Input: part model. Units: mm. Frame: model coordinates. Face numbers are marked on the shaded views. Round coordinates to 2 decimals unless told otherwise and drop trailing zeros. Loops run counter-clockwise (first coordinate to the right, second up) from the corner with the lowest first, then second, coordinate; pieces in that order, holes last. Notation, with made-up numbers: (34.25, -35) -> (63.25, -35) arc R11 cw to (63.25, -30) -> close; hole circle Ø7 at (37.25, 25.5). An arc over 180 degrees is marked (long way). Answer as a JSON object with one key per item and string values. Group by question number.
Item 1: Material intervals for line 1 (X direction, y = 34.5, z = 0); line 2 (X direction, y = 37.5, z = -2); line 3 (Z direction, x = -2.5, y = 18.5), sorted ascending. Write a range as [from, to].
Item 2: Draft query along Z for the marked faces 1, 2, 3 and 4. Return one class per face: released by +Z, released by -Z, zero draft, split by the parting line, or undercut.
Item 3: Pin query (flat end, axial travel): pin 1 (3 mm diameter, centred on x = 11, y = 27.5, fed in from -Z); pin 2 (4 mm diameter, centred on x = -3, y = 31, fed in from +Z); pin 3 (2.5 mm diameter, centred on x = 1.38, z = -12.7, fed in from +Y); pin 4 (1.5 mm diameter, centred on x = 1, y = 36, fed in from +Z). Return the tip coordinate at first contact, or that it passes through.
Item 4: Section query B-B on y = 32. Return loops of the section in (x, z).
Item 5: Section query C-C on x = 8.75. Return loops of the section in (y, z).
Item 6: Section query A-A on z = 12.5. Return loops of the section in (x, y), and give its area (3 significant figures).
Item 7: Section query D-D on z = -4.25. Return loops of the section in (x, y).
from build123d import *

# Parameters (mm, degrees)
SKETCH1_R           = 15
SKETCH1_R_2         = 1.5
BOSS_EXTRUDE1_DEPTH = 31
SKETCH2_R           = 10
SKETCH2_R_2         = 7.5
BOSS_EXTRUDE2_DEPTH = 10


with BuildPart() as part:
    # Sketch1 → Boss-Extrude1 (new body)
    with BuildSketch(Plane(origin=(0, 0, 0), x_dir=(1, 0, 0), z_dir=(0, 1, 0))):
        with Locations(Location((0, 0, 0), (0, 0, 270))):
            Circle(SKETCH1_R)
        with Locations(Location((-12.697691575, 1.377182715, 0), (0, 0, 270))):
            Circle(SKETCH1_R_2, mode=Mode.SUBTRACT)
        with Locations(Location((1.377182715, 12.697691575, 0), (0, 0, 270))):
            Circle(SKETCH1_R_2, mode=Mode.SUBTRACT)
        with Locations(Location((12.697691575, -1.377182715, 0), (0, 0, 270))):
            Circle(SKETCH1_R_2, mode=Mode.SUBTRACT)
        with Locations(Location((-1.377182715, -12.697691575, 0), (0, 0, 270))):
            Circle(SKETCH1_R_2, mode=Mode.SUBTRACT)
    extrude(amount=BOSS_EXTRUDE1_DEPTH)

    # Sketch2 → Boss-Extrude2 (add)
    with BuildSketch(Plane(origin=(0, 31, 0), x_dir=(1, 0, 0), z_dir=(0, 1, 0))):
        with Locations(Location((0, 0, 0), (0, 0, 270))):
            Circle(SKETCH2_R)
        with Locations(Location((0, 0, 0), (0, 0, 270))):
            Circle(SKETCH2_R_2, mode=Mode.SUBTRACT)
    extrude(amount=BOSS_EXTRUDE2_DEPTH)


solid = part.part
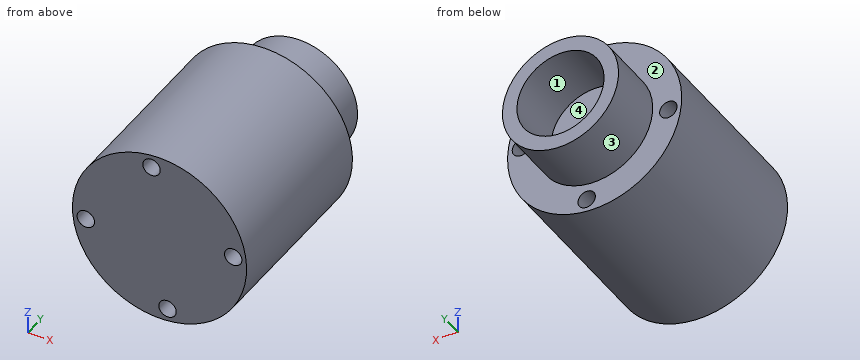
Solved:
{
 "1": {"line 1": "[-10, -7.5], [7.5, 10]", "line 2": "[-9.8, -7.23], [7.23, 9.8]", "line 3": "[-14.79, 11.7], [13.69, 14.79]"},
 "2": {"face 1": "undercut", "face 2": "zero draft", "face 3": "split by the parting line", "face 4": "undercut"},
 "3": {"pin 1": "z = -11.61", "pin 2": "z = 14.97", "pin 3": "through", "pin 4": "z = 10"},
 "4": {"outline": "circle Ø20 at (0, 0); hole circle Ø15 at (0, 0)"},
 "5": {"outline": "(0, -12.18) -> (31, -12.18) -> (31, -4.84) -> (41, -4.84) -> (41, 4.84) -> (31, 4.84) -> (31, 12.18) -> (0, 12.18) -> close"},
 "6": {"outline": "(-8.29, 0) -> (-2.86, 0) -> (-2.86, 31) -> (-8.29, 31) -> close; (0.11, 0) -> (8.29, 0) -> (8.29, 31) -> (0.11, 31) -> close", "area": "422 mm²"},
 "7": {"outline": "(-14.39, 0) -> (14.39, 0) -> (14.39, 31) -> (9.05, 31) -> (9.05, 41) -> (6.18, 41) -> (6.18, 31) -> (-6.18, 31) -> (-6.18, 41) -> (-9.05, 41) -> (-9.05, 31) -> (-14.39, 31) -> close"}
}
